```python
from build123d import *

# Parameters (mm, degrees)
SKETCH1_R           = 3.175
SKETCH1_W           = 14.2875
SKETCH1_H           = 14.2875
BOSS_EXTRUDE1_DEPTH = 1.5875
CUT_EXTRUDE1_DEPTH  = 76.2


with BuildPart() as part:
    # Sketch1 → Boss-Extrude1 (new body)
    with BuildSketch(Plane.XY):
        with BuildLine():
            Line((6.35, 0), (31.75, 0))
            ThreePointArc((31.75, 0), (36.240128061, 1.859871939), (38.1, 6.35))
            Line((38.1, 6.35), (38.1, 69.85))
            ThreePointArc((38.1, 69.85), (36.240128061, 74.340128061), (31.75, 76.2))
            Line((31.75, 76.2), (6.35, 76.2))
            ThreePointArc((6.35, 76.2), (1.859871939, 74.340128061), (0, 69.85))
            Line((0, 69.85), (0, 6.35))
            ThreePointArc((0, 6.35), (1.859871939, 1.859871939), (6.35, 0))
        make_face()
        with Locations((19.05, 38.1)):
            Circle(SKETCH1_R, mode=Mode.SUBTRACT)
        with Locations((19.05, 63.5)):
            Circle(SKETCH1_R, mode=Mode.SUBTRACT)
        with Locations((19.05, 13.49375)):
            Rectangle(SKETCH1_W, SKETCH1_H, mode=Mode.SUBTRACT)
    extrude(amount=BOSS_EXTRUDE1_DEPTH)

    # Sketch3 → Cut-Extrude1 (cut)
    with BuildSketch(Plane.ZY):
        Polygon((0.396875, 0), (1.5875, 1.190625), (1.5875, 0), align=None)
    extrude(amount=-CUT_EXTRUDE1_DEPTH, mode=Mode.SUBTRACT)


solid = part.part
```
Part model, mm, in its own coordinate system. A direction names the side the tool comes from. Round coordinates to 2 decimals unless told otherwise and drop trailing zeros. Write each loop counter-clockwise with the first axis right and the second up, starting at its lowest first coordinate (ties: lowest second). Pieces come first, ordered by that corner, then holes. Notation, with made-up numbers: M -35,-11.75 L -10,-11.75 A10 ccw -10,-4.75 Z; hole C 14.5,14.25 d5. An arc over 180 degrees is marked long. One line per question, with ' | ' between items.
(1) Saw through at A-A on y = 63.5. Write the cut outline in (x, z) (1 decimal).
Answer key:
outline: M 0,0 L 15.9,0 L 15.9,1.6 L 0,1.6 Z; M 22.2,0 L 38.1,0 L 38.1,1.6 L 22.2,1.6 Z
(2) Saw through at D-D on x = 34.5. Write the cut outline in (y, z), then the cut area to 3 significant figures.
Answer key:
outline: M 0.63,0 L 75.57,0 L 75.57,1.59 L 1.19,1.59 L 0.63,1.02 Z | area: 119 mm^2
(3) Two-plate mould, pull along Y, no slides. Class faces 1 (the face through (1.91, 74.39, 0.78)), 2 (the face through (36.91, 2.65, 0.78)), 3 (the face through (19, 6.35, 1)): released by +Y, released by -Y, zero draft, split by the parting line, or undercut.
Answer key:
face 1: released by +Y | face 2: released by -Y | face 3: undercut
(4) Probe line 1 along Y through (x, z) = (17.5, 0.45); line 2 along Y through (x, z) = (20, 0.25); line 3 along X through (y, z) = (12, 1.25). List the from-to ranges inside material, lowest first.
Answer key:
line 1: y = 0.05 to 6.35, 20.64 to 35.33, 40.87 to 60.73, 66.27 to 76.2 | line 2: y = 0 to 6.35, 20.64 to 35.07, 41.13 to 60.47, 66.53 to 76.2 | line 3: x = 0 to 11.91, 26.19 to 38.1
(5) 3-axis set-ups, long thin cutter, end or side, ignore diameter. For faces 4 (the face through (23, 39, 0)), 5 (the face through (19, 20.638, 1)): which of +Z, -Z, +X, -X, +Y, -Y reach the whole face in a straight line?
Answer key:
face 4: -Z, +X, -X, +Y, -Y | face 5: +Z, -Z
(6) Saw through at B-B on x = 19.05. Count the separate pieces of the cut face and the enclosed holes in it, then the cut area to 3 significant figures.
Answer key:
separate pieces: 4 | enclosed holes: 0 | area: 77.4 mm^2
(7) Pin check, flat tips, straight feed: pin 1 (1 mm diameter, centred on x = 22.5, y = 20.5, fed in from -Z); pin 2 (5.5 mm diameter, centred on x = 19.05, y = 63.5, fed in from -Z). Stop position of each tip, or through.
Answer key:
pin 1: stops at z = 0 | pin 2: passes through
